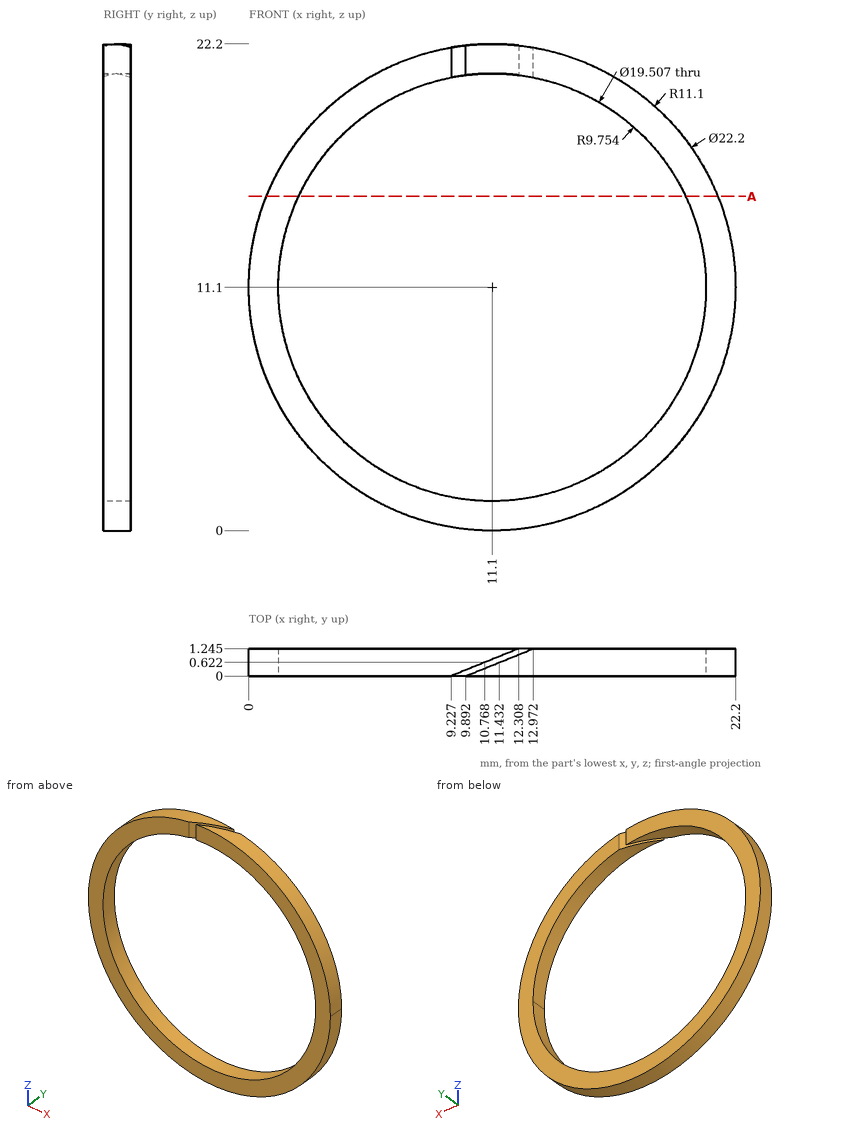
The drawing under review shows one solid part. Ordinate dimensions are in mm from its lowest x, y, z. Coordinates: 2 decimals unless noted, no trailing zeros. Order: outer loops, then holes, each group sorted by start corner. A loop starts at its lowest first (then second) coordinate and runs counter-clockwise, first axis right, second up. Notation, with made-up numbers: (85, -17) -> (127, -17) arc R18 cw to (127, 0) -> close; hole circle Ø2 at (1, 36). An arc over 180 degrees is marked (long way). Return JSON: item names as keys, results as strings.
1. We need section A-A on z = 15.25. Write out the cut boundary in (x, y) (1 decimal).
Answer block:
{"outline": "(0.8, 0) -> (2.3, 0) -> (2.3, 1.2) -> (0.8, 1.2) -> close; (19.9, 0) -> (21.4, 0) -> (21.4, 1.2) -> (19.9, 1.2) -> close"}
2. For pin 1 Ø6 at (x, z) = (14.5, 3.5) entering from +Y (1 decimal); pin 2 Ø1.5 at (x, z) = (9, 19) entering from -Y, all flat-tipped, find the tip position at first contact; note any pin that passes through.
Answer block:
{"pin 1": "y = 1.2", "pin 2": "through"}
3. For line 1 (X direction, y = 0.45, z = 11); line 2 (Z direction, x = 8.5, y = 0.1); line 3 (X direction, y = 0.2, z = 10) (1 decimal), list the stretches that pass through material, from the lowest coordinate up. Write a range as from..to.
Answer block:
{"line 1": "0..1.35, 20.85..22.2", "line 2": "0.31..1.7, 20.5..21.89", "line 3": "0.1..1.4, 20.8..22.1"}
